Autodesk Inventor part; units mm, degrees
ref_plane "YZ Plane" through (0, 0, 0) normal (1, 0, 0) x (0, 1, 0)
ref_plane "XZ Plane" through (0, 0, 0) normal (0, 1, 0) x (-1, 0, 0)
ref_plane "XY Plane" through (0, 0, 0) normal (0, 0, 1) x (1, 0, 0)
sketch "Sketch1" plane through (0, 0, 0) normal (0, 1, 0) x (-1, 0, 0)
  line L0 (0, 0) -> (-76.2, 0)
  line L1 (-76.2, 0) -> (-76.2, -50.8)
  line L2 (-76.2, -50.8) -> (0, -50.8)
  line L3 (0, -50.8) -> (0, 0)
  line L4 (0, -25.4) -> (-76.2, -25.4)
  line L5 (-38.1, -50.8) -> (-38.1, 0)
  line L6 (-6.35, -44.45) -> (-69.85, -44.45) construction
  line L7 (-69.85, -44.45) -> (-69.85, -6.35) construction
  line L8 (-69.85, -6.35) -> (-6.35, -6.35) construction
  line L9 (-6.35, -6.35) -> (-6.35, -44.45) construction
  line L10 (-6.35, -44.45) -> (-69.85, -6.35) construction
  line L11 (-69.85, -44.45) -> (-6.35, -6.35) construction
  circle A0 centre (-6.35, -44.45) radius 1.5875
  circle A1 centre (-69.85, -44.45) radius 1.5875
  circle A2 centre (-6.35, -6.35) radius 1.5875
  circle A3 centre (-69.85, -6.35) radius 1.5875
  circle A4 centre (-38.1, -25.4) radius 4.5
  dimension "d0" = 76.2
  dimension "d1" = 50.8
  dimension "d2" = 63.5
  dimension "d3" = 38.1
  dimension "d4" = 3.175
  dimension "d13" = 9
extrude "Plate1" add sketch "Sketch1" against normal blind 0.9119 contours L3 L4 A4 L5 L0 | L5 A4 L4 L1 L0 | L3 L2 L5 A4 L4 | A4 L4 L5 | L5 L4 A4 | A4 L5 L4 | L4 A4 L5 L2 L1 | L5 A4 L4 | A0 | A1 | A2 | A3
hole "Mounting Holes" at (6.35, 0, -44.45) at (69.85, 0, -44.45) at (69.85, 0, -6.35) at (6.35, 0, -6.35) direction (0, -1, 0) diameter 3.81 end through all countersink diameter 7.0866 countersink angle 82
hole "Input Jack Hole" at (38.1, 0, -25.4) direction (0, -1, 0) diameter 9 end through all
fillet "Corner Round1" radius 3.175 4 edges at (0, -0.4559, -50.8) (76.2, -0.4559, -50.8) (76.2, -0.4559, 0) (0, -0.4559, 0)
equation "\"d11\" = Thickness"
equation "\"d5\" = Thickness"
equation "\"BendRadius\" = Thickness"
equation "\"BendReliefWidth\" = Thickness"
equation "\"BendReliefDepth\" = 0.5 * Thickness"
equation "\"CornerReliefSize\" = 4 * Thickness"
equation "\"MinimumRemnant\" = 2 * Thickness"
equation "\"TransitionRadius\" = BendRadius"
equation "\"JacobiRadiusSize\" = BendRadius"
equation "\"GapSize\" = Thickness"
properties part number "Jack Plate" material "Steel, Carbon"
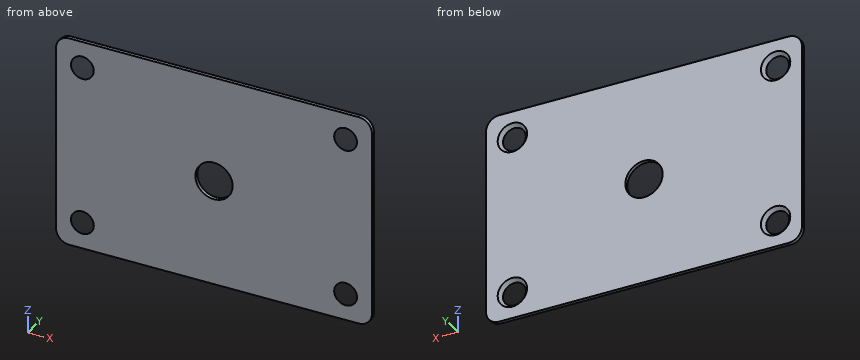
Work out the finished part from the listing and answer in its coordinate system (mm). Coordinates: 2 decimals unless noted, no trailing zeros. Write each loop counter-clockwise with the first axis right and the second up, starting at its lowest first coordinate (ties: lowest second). Pieces come first, ordered by that corner, then holes. Notation, with made-up numbers: M 46,59 L 64,59 A24 cw 64,78 Z; hole C 66.5,-30 d10. An arc over 180 degrees is marked long. Use one line per item in the form item = value. Start each with the question number.
1. The part is cut by section A-A (x = 38.1). Give the vertices of the cut face in (y, z).
2. The part is cut by section D-D (x = 6.35). Give the vertices of the cut face in (y, z).
3. The part is cut by section C-C (y = -0.7). Give the vertices of the cut face in (x, z) (3 decimals), plus the area to 3 significant figures.
4. Straight lines are drawn through the part: probe 1 along Z at (x, y) = (38.1, -0.45); probe 2 along X at (y, z) = (-0.75, -42.5); probe 3 along X at (y, z) = (-0.85, -44). For each, find the intervals that lie inside material, in ascending order. Write a range as from..to.
5. The part is cut by section B-B (z = -28). Give the vertices of the cut face in (x, y).
6. Each of these flat-tipped pins is pushed along its axis until it touches: P1, Ø8, axis at x = 38.1, z = -25.4, coming from the +Y side; P2, Ø1, axis at x = 25, z = -27, coming from the +Y side. Where does it stop, or does it pass through?
Evaluation:
q1.outline = M -0.91,-50.8 L 0,-50.8 L 0,-29.9 L -0.91,-29.9 Z; M -0.91,-20.9 L 0,-20.9 L 0,0 L -0.91,0 Z
q2.outline = M -0.91,-50.8 L 0,-50.8 L 0,-47.99 L -0.91,-47.2 Z; M -0.91,-41.7 L 0,-40.91 L 0,-9.89 L -0.91,-9.1 Z; M -0.91,-3.6 L 0,-2.81 L 0,0 L -0.91,0 Z
q3.outline = M 0,-47.625 A3.175 ccw 3.175,-50.8 L 73.025,-50.8 A3.175 ccw 76.2,-47.625 L 76.2,-3.175 A3.175 ccw 73.025,0 L 3.175,0 A3.175 ccw 0,-3.175 Z; hole C 6.35,-44.45 d5.87; hole C 6.35,-6.35 d5.87; hole C 38.1,-25.4 d9; hole C 69.85,-44.45 d5.87; hole C 69.85,-6.35 d5.87
q3.area = 3,690 mm^2
q4.probe_1 = -50.8..-29.9, -20.9..0
q4.probe_2 = 0..4.22, 8.48..67.72, 71.98..76.2
q4.probe_3 = 0..3.58, 9.12..67.08, 72.62..76.2
q5.outline = M 0,-0.91 L 34.43,-0.91 L 34.43,0 L 0,0 Z; M 41.77,-0.91 L 76.2,-0.91 L 76.2,0 L 41.77,0 Z
q6.P1 = through
q6.P2 = 0
